Design review of the part shown in the three views and the two pictorial views. Dimensions are in mm from the part's minimum x, y and z. Coordinates: 2 decimals unless noted, no trailing zeros. Write each loop counter-clockwise with the first axis right and the second up, starting at its lowest first coordinate (ties: lowest second). Pieces come first, ordered by that corner, then holes. Notation, with made-up numbers: (37, -21.75) - (95, -21.75) arc R7 cw to (95, -12.75) - close; hole circle Ø7 at (-19, -29). An arc over 180 degrees is marked (long way). Write each question's results on one line, items separated by ' | '.
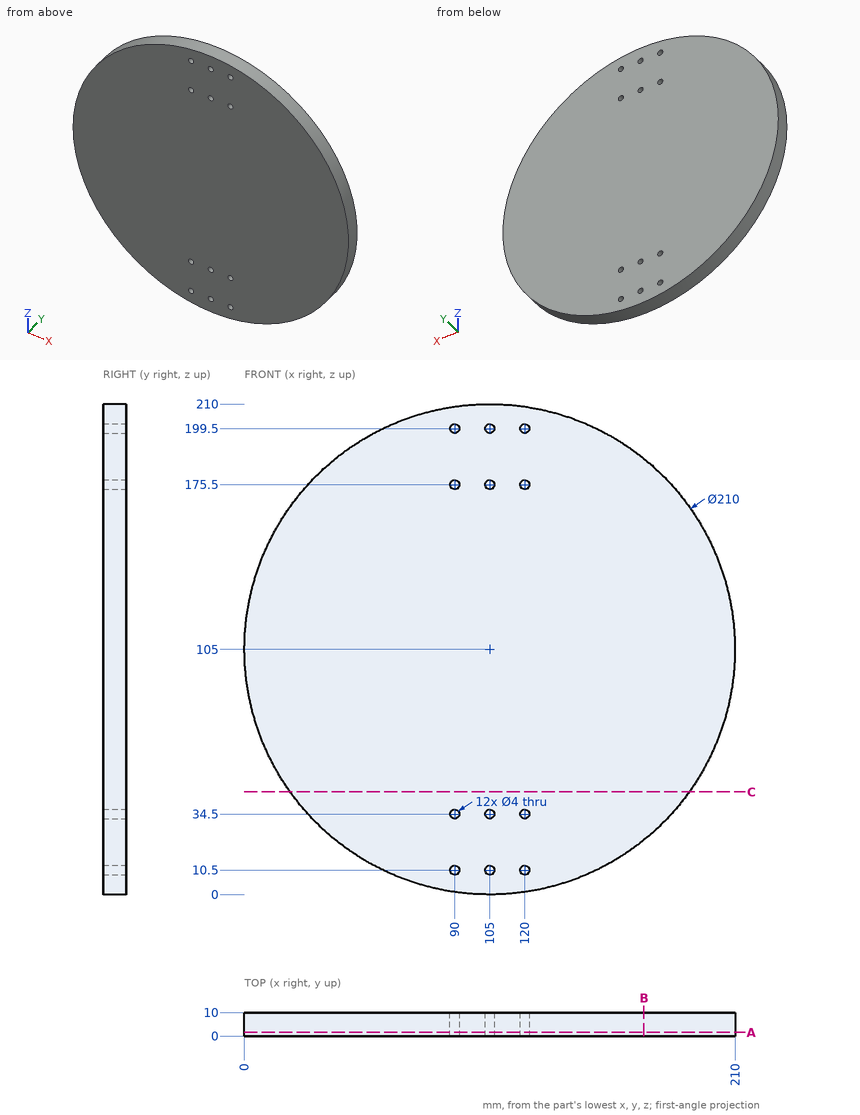
Q1. For pin 1 (3 mm diameter, centred on x = 120, z = 10.5, fed in from +Y); pin 2 (4 mm diameter, centred on y = 5.5, z = 184, fed in from -X); pin 3 (3 mm diameter, centred on y = 7.5, z = 170.5, fed in from -X); pin 4 (6 mm diameter, centred on y = 4, z = 128, fed in from +X), all flat-tipped, find the tip position at first contact; note any pin that passes through.
Results found:
pin 1: through | pin 2: x = 33.61 | pin 3: x = 21.76 | pin 4: x = 208.08
Q2. Wall thickness on line 1 along Z through (x, y) = (105, 6.5); line 2 along Z through (x, y) = (90, 7.5); line 3 along X through (y, z) = (6, 199.5): over which ranges is each line inside the solid? List them lowest first. Write a range as from..to.
Results found:
line 1: 0..8.5, 12.5..32.5, 36.5..173.5, 177.5..197.5, 201.5..210 | line 2: 1.08..8.5, 12.5..32.5, 36.5..173.5, 177.5..197.5, 201.5..208.92 | line 3: 59.23..88, 92..103, 107..118, 122..150.77
Q3. Take a section at C-C on z = 44. State the section outline as (x, y) points.
Results found:
outline: (19.54, 0) - (190.46, 0) - (190.46, 10) - (19.54, 10) - close
Q4. Take a section at B-B on x = 171. State the section outline as (y, z) points, plus the area to 3 significant figures.
Results found:
outline: (0, 23.34) - (10, 23.34) - (10, 186.66) - (0, 186.66) - close | area: 1,630 mm2
Q5. Take a section at A-A on y = 1.5. State how many separate pieces and enclosed holes the cut face has, plus the area to 3 significant figures.
Results found:
separate pieces: 1 | enclosed holes: 12 | area: 34,500 mm2
